```python
from build123d import *


with BuildPart() as part:
    # OutRacSke → OuterRace (revolve)
    with BuildSketch(Plane.XY):
        with BuildLine():
            Line((-3, 19.382436034), (-15, 16.3905))
            Line((-15, 16.3905), (-15, 20.4))
            ThreePointArc((-15, 20.4), (-14.824264069, 20.824264069), (-14.4, 21))
            Line((-14.4, 21), (-3.48, 21))
            Line((-3.48, 21), (-3, 20.52))
            Line((-3, 20.52), (-3, 19.382436034))
        make_face()
    revolve(axis=Axis((-42.5, 0, 0), (1, 0, 0)))

    # RolSimSke → RollersSimplified (revolve)
    with BuildSketch(Plane.XY):
        Polygon((-14.4, 16.622797286), (-3.920806156, 19.235553758), (-2.723292773, 14.432589913), (-13.202486617, 11.81983344), align=None)
    revolve(axis=Axis((0, 0, 0), (-1, 0, 0)))

    # InsRacSke → InnerRace (revolve)
    with BuildSketch(Plane.XY):
        with BuildLine():
            Line((-13.258207732, 12.06733344), (-15, 12.06733344))
            Line((-15, 12.06733344), (-15, 10.48))
            Line((-15, 10.48), (-14.52, 10))
            Line((-14.52, 10), (-0.6, 10))
            ThreePointArc((-0.6, 10), (-0.175735931, 10.175735931), (0, 10.6))
            Line((0, 10.6), (0, 14.927589913))
            Line((0, 14.927589913), (-2.717305207, 14.927589913))
            Line((-2.717305207, 14.927589913), (-2.717305207, 14.432589913))
            Line((-2.717305207, 14.432589913), (-13.196499051, 11.81983344))
            Line((-13.196499051, 11.81983344), (-13.258207732, 12.06733344))
        make_face()
    revolve(axis=Axis((-42.5, 0, 0), (1, 0, 0)))


solid = part.part
```
Check sheet for the modelled part. Datum: model origin and axes. Units: mm. A direction names the side the tool comes from. Coordinates: 2 decimals unless noted, no trailing zeros. Loops run counter-clockwise (first coordinate to the right, second up) from the corner with the lowest first, then second, coordinate; pieces in that order, holes last. Notation, with made-up numbers: M 28,-10.5 L 79,-10.5 A23 ccw 79,12.5 Z; hole C 31.5,82 d2. An arc over 180 degrees is marked long. Answer as a JSON object with one key per item and string values.
1. Access from +Z, -Z, +X, -X, +Y, -Y to the whole of each face (thin tool, end or side, straight path). Record for faces 1 (the cylindrical face through (-14.14, -9.58, -7.34)), 2 (the flat face through (-3, 8, -18)), 3 (the flat face through (0, 4, 10)).
Outcome:
{"face 1": "-X", "face 2": "+X", "face 3": "+Z, -Z, +X, +Y, -Y"}
2. Sectioned sample at B-B on x = -1.5. Record the cut outline in (y, z).
Outcome:
{"outline": "C 0,0 d29.86; hole C 0,0 d20"}
3. Sectioned sample at A-A on x = -12.25. Record the cut outline in (y, z).
Outcome:
{"outline": "C 0,0 d42; C 0,0 d24.11; hole C 0,0 d24.11; hole C 0,0 d20"}
4. Depth check by flat-ended pin: P1, Ø2, axis at x = -10, y = -10, coming from the -Z side; P2, Ø9, axis at y = -2.5, z = -2, coming from the -X side; P3, Ø1, axis at x = -5, y = -14, coming from the -Z side; P4, Ø2, axis at y = -13.5, z = 15, coming from the +X side. Enter the tip coordinate at first touch or a pass-through.
Outcome:
{"P1": "z = -18.97", "P2": "through", "P3": "z = -16.09", "P4": "x = -3"}
5. Sectioned sample at C-C on x = -8.75. Record the cut outline in (y, z).
Outcome:
{"outline": "C 0,0 d42; C 0,0 d25.86; hole C 0,0 d25.86; hole C 0,0 d20"}
6. Scan lines: L1, parallel to Y at x = -1, z = 6; L2, parallel to X at y = 10.5, z = -1; L3, parallel to Y at x = -11.5, z = -16. Record each from-to range of solid material in increasing order. Write a range as from..to.
Outcome:
{"L1": "-13.67..-8, 8..13.67", "L2": "-15..0", "L3": "-13.6..13.6"}
